Check sheet for the modelled part. Datum: model origin and axes. Units: mm. A direction names the side the tool comes from. Round coordinates to 2 decimals unless told otherwise and drop trailing zeros. Loops run counter-clockwise (first coordinate to the right, second up) from the corner with the lowest first, then second, coordinate; pieces in that order, holes last. Notation, with made-up numbers: (-36, -21.5) - (-9, -21.5) arc R22 cw to (-9, 0.5) - close; hole circle Ø10 at (13, -22). An arc over 180 degrees is marked (long way). Put each result on its own line as item: value. Start each with the question number.
Item 1: Material ranges on line 1 along Y through (x, z) = (-1.9, 18.05); line 2 along Y through (x, z) = (0.25, 19.25); line 3 along X through (y, z) = (-16, 12.5), recorded low to high.
Item 2: Section check B-B, the plane x = 0. Give the number of separate pieces and of enclosed holes in the cut face, and give its area (3 significant figures).
Item 3: Section check C-C, the plane y = -22. Record the cut outline in (x, z).
Item 4: Tool access check on faces 1 (the flat face through (3, 0, 14)), 2 (the flat face through (4.874, 22.771, 9.86)), 3 (the flat face through (5, 15, 15.5)). Record the directions out of +Z, -Z, +X, -X, +Y, -Y that give a thin tool (end or side, any length) a straight path to the whole face; none if there is none.
Item 5: Section check A-A, the plane z = 16.75. Record the cut outline in (x, y), and give its area (3 significant figures).
Item 6: Gauge pin test, flat ends, axial feed: pin 1 Ø3 at (x, z) = (2.5, 4) entering from +Y; pin 2 Ø3 at (x, z) = (-1, 16) entering from -Y; pin 3 Ø2 at (x, y) = (0, -23.75) entering from +Z; pin 4 Ø2 at (x, z) = (4.5, 14.5) entering from +Y. Record the tip position at first contact, or that the pin passes through.
Item 7: Draft check along X on faces 4 (the cylindrical face through (0, -25, 10)), 5 (the flat face through (-8, 0, 10)), 6 (the flat face through (8, 0, 10)), 7 (the flat face through (0, -16.25, 14)). Enter one of: pulls with the +X half, pulls with the -X half, needs draft (parallel to the pull), parting line crosses it, or undercut.
from build123d import *

# Parameters (mm, degrees)
F0_R     = 1.25
F1_DEPTH = 20
F2_W     = 14
F2_H     = 38
F2_W_2   = 6
F2_H_2   = 33.5
F3_DEPTH = 12.7
F8_R     = 0.9
F9_DEPTH = 4.5


with BuildPart() as f1:
    # F0 (on Top) → F1 (new body)
    with BuildSketch(Plane.XY):
        Polygon((8, 20), (-8, 20), (-8, 0), (-8, -20), (8, -20), (8, 0), align=None)
        Polygon((-7, 0), (-7, 19), (7, 19), (7, 0), (7, -19), (-7, -19), align=None, mode=Mode.SUBTRACT)
        with BuildLine():
            Line((-1.6582336623, 25.6208984796), (-8, 20))
            Line((-8, 20), (8, 20))
            Line((8, 20), (1.6582336623, 25.6208984796))
            ThreePointArc((1.6582336623, 25.6208984796), (2.2798666799, 24.7757718665), (2.5, 23.75))
            ThreePointArc((2.5, 23.75), (-1.0257718665, 21.4701333201), (-1.6582336623, 25.6208984796))
        make_face()
        with BuildLine():
            ThreePointArc((1.6582336623, 25.6208984796), (0, 26.25), (-1.6582336623, 25.6208984796))
            ThreePointArc((-1.6582336623, 25.6208984796), (-1.0257718665, 21.4701333201), (2.5, 23.75))
            ThreePointArc((2.5, 23.75), (2.2798666799, 24.7757718665), (1.6582336623, 25.6208984796))
        make_face()
        with Locations((0, 23.75)):
            Circle(F0_R, mode=Mode.SUBTRACT)
        with BuildLine():
            Line((8, -20), (-8, -20))
            Line((-8, -20), (-1.6582336623, -25.6208984796))
            ThreePointArc((-1.6582336623, -25.6208984796), (-1.0257718665, -21.4701333201), (2.5, -23.75))
            ThreePointArc((2.5, -23.75), (2.2798666799, -24.7757718665), (1.6582336623, -25.6208984796))
            Line((1.6582336623, -25.6208984796), (8, -20))
        make_face()
        with BuildLine():
            ThreePointArc((2.5, -23.75), (-1.0257718665, -21.4701333201), (-1.6582336623, -25.6208984796))
            ThreePointArc((-1.6582336623, -25.6208984796), (0, -26.25), (1.6582336623, -25.6208984796))
            ThreePointArc((1.6582336623, -25.6208984796), (2.2798666799, -24.7757718665), (2.5, -23.75))
        make_face()
        with Locations((0, -23.75)):
            Circle(F0_R, mode=Mode.SUBTRACT)
    extrude(amount=F1_DEPTH)

    # F2 (on face) → F3 (join)
    with BuildSketch(Plane.XY.offset(20)):
        Rectangle(F2_W, F2_H)
        with Locations((0, 0.5)):
            Rectangle(F2_W_2, F2_H_2, mode=Mode.SUBTRACT)
    extrude(amount=-F3_DEPTH)

    # F6: sweep along a path in F6_path
    with BuildLine(Plane(origin=(-7, 19, 0), x_dir=(0, 1, 0), z_dir=(0, 0, 1))) as f6_path:
        Line((0, 0), (0, -14))
    # F4 (on face) → F6 (sweep)
    with BuildSketch(Plane.YZ.offset(-7)):
        with BuildLine():
            Line((-19, 7.3), (-19, 0))
            add(Edge.make_bspline(
                [(-19, 0), (-16.966280043, 0), (-16.25, 4.7682679952), (-16.25, 7.3)],
                knots=[0, 0, 0, 0, 7.8008012409, 7.8008012409, 7.8008012409, 7.8008012409], degree=3))
            Line((-16.25, 7.3), (-19, 7.3))
        make_face()
        with BuildLine():
            Line((19, 7.3), (17.25, 7.3))
            add(Edge.make_bspline(
                [(19, 0), (16.966280043, 0), (17.25, 4.7682679952), (17.25, 7.3)],
                knots=[0, 0, 0, 0, 7.5068302232, 7.5068302232, 7.5068302232, 7.5068302232], degree=3))
            Line((19, 0), (19, 7.3))
        make_face()
    sweep(path=f6_path.line)

    # F7: sweep along a path in F7_path
    with BuildLine(Plane(origin=(-7, -19, 0), x_dir=(0, -1, 0), z_dir=(0, 0, -1))) as f7_path:
        Line((0, 0), (-38, 0))
    # F5 (on face) → F7 (sweep)
    with BuildSketch(Plane(origin=(0, -19, 0), x_dir=(-1, 0, 0), z_dir=(0, 1, 0))):
        with BuildLine():
            add(Edge.make_bspline(
                [(7, 0), (4.5295656249, 0), (3, 4.5769013319), (3, 7.3)],
                knots=[0, 0, 0, 0, 8.3240615087, 8.3240615087, 8.3240615087, 8.3240615087], degree=3))
            Line((7, 0), (7, 7.3))
            Line((7, 7.3), (3, 7.3))
        make_face()
        with BuildLine():
            Line((-7, 7.3), (-7, 0))
            add(Edge.make_bspline(
                [(-7, 0), (-4.5295656249, 0), (-3, 4.5769013319), (-3, 7.3)],
                knots=[0, 0, 0, 0, 8.3240615087, 8.3240615087, 8.3240615087, 8.3240615087], degree=3))
            Line((-3, 7.3), (-7, 7.3))
        make_face()
    sweep(path=f7_path.line)

    # F8 (on face) → F9 (cut)
    with BuildSketch(Plane.XY.offset(20)):
        with Locations((5.5, 14.94)):
            Circle(F8_R)
        with Locations((-1.9, -17.95)):
            Circle(F8_R)
    extrude(amount=-F9_DEPTH, mode=Mode.SUBTRACT)


solid = f1.part
Check result:
1. line 1: -25.41 to -18.85, -17.05 to -16.25, 17.25 to 25.41
1. line 2: -26.24 to -24.97, -22.53 to -16.25, 17.25 to 22.53, 24.97 to 26.24
1. line 3: -8 to -3, 3 to 8
2. separate pieces: 4
2. enclosed holes: 0
2. area: 274 mm²
3. outline: (-5.74, 0) - (5.74, 0) - (5.74, 20) - (-5.74, 20) - close
4. face 1: +Z, -Z
4. face 2: +Z, -Z, +X, +Y
4. face 3: +Z
5. outline: (-8, -20) - (-1.66, -25.62) arc R2.5 ccw to (1.66, -25.62) - (8, -20) - (8, 20) - (1.66, 25.62) arc R2.5 ccw to (-1.66, 25.62) - (-8, 20) - close; hole (-3, -16.25) - (3, -16.25) - (3, 17.25) - (-3, 17.25) - close; hole circle Ø1.8 at (-1.9, -17.95); hole circle Ø2.5 at (0, -23.75); hole circle Ø2.5 at (0, 23.75); hole circle Ø1.8 at (5.5, 14.94)
5. area: 536 mm²
6. pin 1: y = 26.04
6. pin 2: y = -26.25
6. pin 3: through
6. pin 4: y = 23.99
7. face 4: undercut
7. face 5: pulls with the -X half
7. face 6: pulls with the +X half
7. face 7: undercut
